```python
from build123d import *

# Parameters (mm, degrees)
SKETCH1_R                    = 2.5
BASE_FLANGE3_DEPTH           = 0.7366
SKETCHED_START               = -64
SKETCHED_BEND1_OUTLINE_W     = 0.7366
SKETCHED_BEND1_OUTLINE_H     = 65
SKETCHED_BEND1_DEPTH         = 64.108877104
SKETCHED_START_2             = 0.168203781
SKETCHED_BEND1_2_DEPTH       = 0.525916755
SKETCHED_START_3             = -0.042479464
SKETCHED_BEND1_3_DEPTH       = 1.4732
SKETCHED_START_4             = -32.5
SKETCHED_BEND1_4_DEPTH       = 65
EDGE_FLANGE1_START           = 0.7366
EDGE_FLANGE1_DEPTH           = 30.75756821
EDGE_FLANGE1_START_2         = 31.12586821
EDGE_FLANGE1_2_DEPTH         = 0.3683
EDGE_FLANGE1_3_DEPTH         = 30.38926821
SKETCH19_R                   = 1.27
SKETCH19_R_2                 = 3.3749
CUT_EXTRUDE5_DEPTH           = 112.820280988
SKETCH20_W                   = 42.572846016
SKETCH20_H                   = 16.402646855
CUT_EXTRUDE6_DEPTH           = 98.335621766
EDGE_FLANGE2_START           = 0.7366
EDGE_FLANGE2_DEPTH           = 30.75756821
EDGE_FLANGE2_START_2         = 31.12586821
EDGE_FLANGE2_2_DEPTH         = 0.3683
EDGE_FLANGE2_3_DEPTH         = 30.38926821
SKETCH27_R                   = 2.575
CUT_EXTRUDE7_DEPTH           = 10
CUT_EXTRUDE8_DEPTH           = 98.335621766
CUT_EXTRUDE8_DEPTH_BACK      = 98.335621766
SKETCH28_R                   = 1.725
SKETCH33_W                   = 30
SKETCH33_H                   = 65
SKETCH33_R                   = 2
TAB1_DEPTH                   = 0.7366
EDGE_FLANGE3_STRIP_W         = 4.4196
EDGE_FLANGE3_STRIP_H         = 0.7366
EDGE_FLANGE3_STRIP_CUT_DEPTH = 59.2634
EDGE_FLANGE3_DEPTH           = 59.2634
EDGE_FLANGE4_STRIP_W         = 4.4196
EDGE_FLANGE4_STRIP_H         = 0.7366
EDGE_FLANGE4_STRIP_CUT_DEPTH = 59.2634
EDGE_FLANGE4_DEPTH           = 59.2634


with BuildPart() as part:
    # Base-Flange3: sheet metal written as solids
    # Sketch1 → Base-Flange3 (new body)
    with BuildSketch(Plane(origin=(0, 0, 0), x_dir=(1, 0, 0), z_dir=(0, 1, 0))):
        with BuildLine():
            Line((-30.694120536, 32.5), (30.694120536, 32.5))
            Line((30.694120536, 32.5), (30.694120536, -32.5))
            Line((30.694120536, -32.5), (-30.694120536, -32.5))
            ThreePointArc((-30.694120536, -32.5), (-63.194120536, 0), (-30.694120536, 32.5))
        make_face()
        with Locations(Location((15.694120536, 0, 0), (0, 0, 270))):
            Circle(SKETCH1_R, mode=Mode.SUBTRACT)
    extrude(amount=-BASE_FLANGE3_DEPTH)

    # Sketched Bend1: read off the stored shape, not the designer's step
    # Sketched Bend1 outline → Sketched Bend1 (cut)
    with BuildSketch(Plane.YZ.offset(SKETCHED_START)):
        with Locations((-0.3683, 0)):
            Rectangle(SKETCHED_BEND1_OUTLINE_W, SKETCHED_BEND1_OUTLINE_H)
    extrude(amount=SKETCHED_BEND1_DEPTH, mode=Mode.SUBTRACT)

    # Sketched Bend1 2 outline → Sketched Bend1 2 (add)
    with BuildSketch(Plane.YZ.offset(SKETCHED_START_2)):
        with BuildLine():
            ThreePointArc((31.12586821, -32.5), (63.62586821, 0), (31.12586821, 32.5))
            Line((31.12586821, 32.5), (0, 32.5))
            Line((0, 32.5), (0, -32.5))
            Line((0, -32.5), (31.12586821, -32.5))
        make_face()
    extrude(amount=SKETCHED_BEND1_2_DEPTH)

    # Sketched Bend1 3 outline → Sketched Bend1 3 (add)
    with BuildSketch(Plane.YZ.offset(SKETCHED_START_3)):
        with BuildLine():
            ThreePointArc((31.12586821, -32.5), (63.62586821, 0), (31.12586821, 32.5))
            Line((31.12586821, 32.5), (0, 32.5))
            Line((0, 32.5), (0, -32.5))
            Line((0, -32.5), (31.12586821, -32.5))
        make_face()
    extrude(amount=SKETCHED_BEND1_3_DEPTH)

    # Sketched Bend1 4 outline → Sketched Bend1 4 (cut)
    with BuildSketch(Plane.XY.offset(SKETCHED_START_4)):
        with BuildLine():
            Line((0.694120536, 65), (0.694120536, 0.7366))
            ThreePointArc((0.694120536, 0.7366), (0.90986568, 0.215745144), (1.430720536, 0))
            Line((1.430720536, 0), (1.430720536, 65))
            Line((1.430720536, 65), (0.694120536, 65))
        make_face()
        with BuildLine():
            Line((-0.042479464, 0.7366), (-0.042479396, 65))
            Line((-0.042479396, 65), (-2, 65))
            Line((-2, 65), (-2, 0))
            Line((-2, 0), (0.108877104, 0))
            Line((0.108877104, 0), (0.108877104, -2))
            Line((0.108877104, -2), (32, -2))
            Line((32, -2), (32, -0.736599968))
            Line((32, -0.736599968), (1.430720536, -0.7366))
            ThreePointArc((1.430720536, -0.7366), (0.389010825, -0.30510971), (-0.042479464, 0.7366))
        make_face()
    extrude(amount=SKETCHED_BEND1_4_DEPTH, mode=Mode.SUBTRACT)

    # Edge-Flange1: read off the stored shape, not the designer's step
    # Edge-Flange1 outline → Edge-Flange1 (cut)
    with BuildSketch(Plane(origin=(0, 0, 0), x_dir=(1, 0, 0), z_dir=(0, 1, 0)).offset(EDGE_FLANGE1_START)):
        with BuildLine():
            ThreePointArc((0.496749161, 32.5), (0.643922463, 32.144692217), (0.694120536, 31.7634))
            Line((0.694120536, 31.7634), (0.694120536, 32.5))
            Line((0.694120536, 32.5), (0.496749161, 32.5))
        make_face()
    extrude(amount=EDGE_FLANGE1_DEPTH, mode=Mode.SUBTRACT)

    # Edge-Flange1 2 outline → Edge-Flange1 2 (cut)
    with BuildSketch(Plane(origin=(0, 0, 0), x_dir=(1, 0, 0), z_dir=(0, 1, 0)).offset(EDGE_FLANGE1_START_2)):
        with BuildLine():
            Line((-0.042479464, 31.3951), (0.694120536, 31.3951))
            Line((0.694120536, 31.3951), (0.694120536, 31.7634))
            ThreePointArc((0.694120536, 31.7634), (0.643922463, 32.144692217), (0.496749161, 32.5))
            Line((0.496749161, 32.5), (-0.042479464, 32.5))
            Line((-0.042479464, 32.5), (-0.042479464, 31.3951))
        make_face()
    extrude(amount=EDGE_FLANGE1_2_DEPTH, mode=Mode.SUBTRACT)

    # Edge-Flange1 3 outline → Edge-Flange1 3 (add)
    with BuildSketch(Plane(origin=(0, 0, 0), x_dir=(1, 0, 0), z_dir=(0, 1, 0)).offset(EDGE_FLANGE1_START)):
        with BuildLine():
            ThreePointArc((-0.779079464, 32.5), (-0.258224609, 32.284254855), (-0.042479464, 31.7634))
            Line((-0.042479464, 31.7634), (-0.042479464, 32.5))
            Line((-0.042479464, 32.5), (0.496749161, 32.5))
            ThreePointArc((0.496749161, 32.5), (-0.042479464, 33.039228625), (-0.779079464, 33.2366))
            Line((-0.779079464, 33.2366), (-65.042479464, 33.2366))
            Line((-65.042479464, 33.2366), (-65.042479464, 32.5))
            Line((-65.042479464, 32.5), (-0.779079464, 32.5))
        make_face()
    extrude(amount=EDGE_FLANGE1_3_DEPTH)

    # Sketch19 → Cut-Extrude5 (cut, through all)
    with BuildSketch(Plane.XY.offset(-32.5)):
        with Locations((-24.096722092, 26.469477583)):
            Circle(SKETCH19_R)
        with Locations((-9.310652066, 7.044552475)):
            Circle(SKETCH19_R)
        with Locations((-4.517479464, 16.06042365)):
            Circle(SKETCH19_R_2)
    extrude(amount=-CUT_EXTRUDE5_DEPTH, mode=Mode.SUBTRACT)

    # Sketch20 → Cut-Extrude6 (cut, through all)
    with BuildSketch(Plane(origin=(0.694120536, 0, 0), x_dir=(0, 0, -1), z_dir=(1, 0, 0))):
        with Locations((5.381444798, 16.092801871)):
            Rectangle(SKETCH20_W, SKETCH20_H)
    extrude(amount=-CUT_EXTRUDE6_DEPTH, mode=Mode.SUBTRACT)

    # Edge-Flange2: read off the stored shape, not the designer's step
    # Edge-Flange2 outline → Edge-Flange2 (cut)
    with BuildSketch(Plane(origin=(0, 0, 0), x_dir=(1, 0, 0), z_dir=(0, 1, 0)).offset(EDGE_FLANGE2_START)):
        with BuildLine():
            ThreePointArc((0.694120536, -31.7634), (0.643922463, -32.144692217), (0.496749161, -32.5))
            Line((0.496749161, -32.5), (0.694120536, -32.5))
            Line((0.694120536, -32.5), (0.694120536, -31.7634))
        make_face()
    extrude(amount=EDGE_FLANGE2_DEPTH, mode=Mode.SUBTRACT)

    # Edge-Flange2 2 outline → Edge-Flange2 2 (cut)
    with BuildSketch(Plane(origin=(0, 0, 0), x_dir=(1, 0, 0), z_dir=(0, 1, 0)).offset(EDGE_FLANGE2_START_2)):
        with BuildLine():
            Line((-0.042479464, -31.3951), (-0.042479464, -32.5))
            Line((-0.042479464, -32.5), (0.496749161, -32.5))
            ThreePointArc((0.496749161, -32.5), (0.643922463, -32.144692217), (0.694120536, -31.7634))
            Line((0.694120536, -31.7634), (0.694120536, -31.3951))
            Line((0.694120536, -31.3951), (-0.042479464, -31.3951))
        make_face()
    extrude(amount=EDGE_FLANGE2_2_DEPTH, mode=Mode.SUBTRACT)

    # Edge-Flange2 3 outline → Edge-Flange2 3 (add)
    with BuildSketch(Plane(origin=(0, 0, 0), x_dir=(1, 0, 0), z_dir=(0, 1, 0)).offset(EDGE_FLANGE2_START)):
        with BuildLine():
            Line((-0.779079464, -32.5), (-65.042479464, -32.5))
            Line((-65.042479464, -32.5), (-65.042479464, -33.2366))
            Line((-65.042479464, -33.2366), (-0.779079464, -33.2366))
            ThreePointArc((-0.779079464, -33.2366), (-0.042479464, -33.039228625), (0.496749161, -32.5))
            Line((0.496749161, -32.5), (-0.042479464, -32.5))
            Line((-0.042479464, -32.5), (-0.042479464, -31.7634))
            ThreePointArc((-0.042479464, -31.7634), (-0.258224609, -32.284254855), (-0.779079464, -32.5))
        make_face()
    extrude(amount=EDGE_FLANGE2_3_DEPTH)

    # Sketch27 → Cut-Extrude7 (cut)
    with BuildSketch(Plane.XY.offset(38.8834)):
        with Locations((-4.517479464, 16.06042365)):
            Circle(SKETCH27_R)
    extrude(amount=-CUT_EXTRUDE7_DEPTH, mode=Mode.SUBTRACT)

    # Sketch28 → Cut-Extrude8 (cut, two sides: drawn at the far end of the back side and taken through both)
    with BuildSketch(Plane(origin=(0.694120536, 0, 0), x_dir=(0, 0, -1), z_dir=(1, 0, 0)).offset(-CUT_EXTRUDE8_DEPTH_BACK)):
        with Locations(Location((-5.239369246, 44.083803898, 0), (0, 0, 270))):
            Circle(SKETCH28_R)
    extrude(amount=CUT_EXTRUDE8_DEPTH + CUT_EXTRUDE8_DEPTH_BACK, mode=Mode.SUBTRACT)

    # Tab1: sheet metal written as solids
    # Sketch33 → Tab1 (add)
    with BuildSketch(Plane(origin=(0, 0, 0), x_dir=(1, 0, 0), z_dir=(0, 1, 0))):
        with Locations((45.694120536, 0)):
            Rectangle(SKETCH33_W, SKETCH33_H)
        with Locations(Location((45.694120536, 17.5, 0), (0, 0, 270))):
            Circle(SKETCH33_R, mode=Mode.SUBTRACT)
        with Locations(Location((45.694120536, -17.5, 0), (0, 0, 270))):
            Circle(SKETCH33_R, mode=Mode.SUBTRACT)
    extrude(amount=-TAB1_DEPTH)

    # Edge-Flange3: sheet metal written as solids
    # Edge-Flange3 strip (on a plane across the edge) → Edge-Flange3 strip cut (cut)
    with BuildSketch(Plane(origin=(1.430720536, 0, 32.5), x_dir=(0, 0, -1), z_dir=(1, 0, 0))):
        with Locations((-0.7366, -0.3683)):
            Rectangle(EDGE_FLANGE3_STRIP_W, EDGE_FLANGE3_STRIP_H)
    extrude(amount=EDGE_FLANGE3_STRIP_CUT_DEPTH, mode=Mode.SUBTRACT)

    # Edge-Flange3 section (on a plane across the edge) → Edge-Flange3 (add)
    with BuildSketch(Plane(origin=(1.430720536, 0, 32.5), x_dir=(0, 0, -1), z_dir=(1, 0, 0))):
        with BuildLine():
            Line((0, 0.7366), (0, 30.39))
            Line((0, 30.39), (0.7366, 30.39))
            Line((0.7366, 30.39), (0.7366, 0.7366))
            ThreePointArc((0.7366, 0.7366), (0.952345145, 0.215745145), (1.4732, 0))
            Line((1.4732, 0), (1.4732, -0.7366))
            ThreePointArc((1.4732, -0.7366), (0.43149029, -0.30510971), (0, 0.7366))
        make_face()
    extrude(amount=EDGE_FLANGE3_DEPTH)

    # Edge-Flange4: sheet metal written as solids
    # Edge-Flange4 strip (on a plane across the edge) → Edge-Flange4 strip cut (cut)
    with BuildSketch(Plane(origin=(60.694120536, 0, -32.5), x_dir=(0, 0, 1), z_dir=(-1, 0, 0))):
        with Locations((-0.7366, -0.3683)):
            Rectangle(EDGE_FLANGE4_STRIP_W, EDGE_FLANGE4_STRIP_H)
    extrude(amount=EDGE_FLANGE4_STRIP_CUT_DEPTH, mode=Mode.SUBTRACT)

    # Edge-Flange4 section (on a plane across the edge) → Edge-Flange4 (add)
    with BuildSketch(Plane(origin=(60.694120536, 0, -32.5), x_dir=(0, 0, 1), z_dir=(-1, 0, 0))):
        with BuildLine():
            Line((0, 0.7366), (0, 29.6534))
            Line((0, 29.6534), (0.7366, 29.6534))
            Line((0.7366, 29.6534), (0.7366, 0.7366))
            ThreePointArc((0.7366, 0.7366), (0.952345145, 0.215745145), (1.4732, 0))
            Line((1.4732, 0), (1.4732, -0.7366))
            ThreePointArc((1.4732, -0.7366), (0.43149029, -0.30510971), (0, 0.7366))
        make_face()
    extrude(amount=EDGE_FLANGE4_DEPTH)


solid = part.part
```
For this review, take the finished solid that the model builds, in its own axes (mm). A direction names the side the tool comes from. Round coordinates to 2 decimals unless told otherwise and drop trailing zeros. Write each loop counter-clockwise with the first axis right and the second up, starting at its lowest first coordinate (ties: lowest second). Pieces come first, ordered by that corner, then holes. Notation, with made-up numbers: (22.25, 60.5) -> (29.25, 60.5) arc R24 ccw to (29.25, 84.5) -> close; hole circle Ø5 at (-29.5, 47.5). An arc over 180 degrees is marked (long way). One line per question, with ' | ' between items. Start each with the question number.
(1) Add section B-B, the plane y = 21. Write out the cut boundary in (x, z).
(2) Add section D-D, the plane z = -13. Write out the cut boundary in (x, y), plus the area to 3 significant figures.
(3) Add section A-A, the plane z = 0. Write out the cut boundary in (x, y), plus the area to 3 significant figures.
(4) Mouldability with a two-part tool opening along Y and no side actions: class faces 1 (the face through (-2.14, 15.07, 32.87)), 2 (the face through (31, 15, -31.763)), 3 (the face through (31, -0.737, 0)) as released by +Y, released by -Y, zero draft, split by the parting line, or undercut.
(5) Insertion check: P1, Ø1.2, axis at x = -30.5, z = 32.5, coming from the -Y side; P2, Ø1.5, axis at y = 52.5, z = -24.5, coming from the +X side; P3, Ø3, axis at y = 55.5, z = 4.5, coming from the -X side; P4, Ø3, axis at y = 44.08, z = 5.24, coming from the +X side. Each pin has a flat end and moves straight along its axis. Give the tip position at first contact, or say it passes through.
(6) For line 1 along X through (y, z) = (-0.4, -17.5); line 2 along Z through (x, y) = (-36, 29); line 3 along Z through (x, y) = (1.5, 9), list the stretches that pass through material, from the lowest coordinate up. Write a range as from..to.
(7) Add section C-C, the plane x = 52. Write out the cut boundary in (y, z), plus the area to 3 significant figures.
(8) Tool access review of faces 4 (the face through (-33, 16, -32.5)), 5 (the face through (31, 15, 32.5)), 6 (the face through (-24.37, 25.23, -32.86)), 7 (the face through (31, 0, 0)), 8 (the face through (31, 15, -32.5)): name each direction out of +Z, -Z, +X, -X, +Y, -Y from which nothing blocks a thin tool from reaching the whole face with its end or side.
Answer list:
1) outline: (-65.04, -33.24) -> (-0.78, -33.24) arc R1.47 ccw to (0.69, -31.76) -> (0.69, -26.67) -> (-0.04, -26.67) -> (-0.04, -31.76) arc R0.74 cw to (-0.78, -32.5) -> (-65.04, -32.5) -> close; (-65.04, 32.5) -> (-0.78, 32.5) arc R0.74 cw to (-0.04, 31.76) -> (-0.04, 15.9) -> (0.69, 15.9) -> (0.69, 31.76) arc R1.47 ccw to (-0.78, 33.24) -> (-65.04, 33.24) -> close; (1.43, -32.5) -> (60.69, -32.5) -> (60.69, -31.76) -> (1.43, -31.76) -> close; (1.43, 31.76) -> (60.69, 31.76) -> (60.69, 32.5) -> (1.43, 32.5) -> close
2) outline: (-0.04, 0.74) arc R1.47 ccw to (1.43, -0.74) -> (60.69, -0.74) -> (60.69, 0) -> (1.43, 0) arc R0.74 cw to (0.69, 0.74) -> (0.69, 7.89) -> (-0.04, 7.89) -> close; (-0.04, 24.29) -> (0.69, 24.29) -> (0.69, 60.91) -> (-0.04, 60.91) -> close | area: 77.2 mm²
3) outline: (-0.04, 0.74) arc R1.47 ccw to (1.43, -0.74) -> (13.19, -0.74) -> (13.19, 0) -> (1.43, 0) arc R0.74 cw to (0.69, 0.74) -> (0.69, 7.89) -> (-0.04, 7.89) -> close; (-0.04, 24.29) -> (0.69, 24.29) -> (0.69, 63.63) -> (-0.04, 63.63) -> close; (18.19, -0.74) -> (60.69, -0.74) -> (60.69, 0) -> (18.19, 0) -> close | area: 75.5 mm²
4) face 1: undercut | face 2: zero draft | face 3: released by -Y
5) P1: y = 0.74 | P2: x = 0.69 | P3: x = -0.04 | P4: through
6) line 1: 0.49..43.69, 47.69..60.69 | line 2: -33.24..-32.5, 32.5..33.24 | line 3: -32.5..-31.76, 31.76..32.5
7) outline: (-0.74, -31.03) arc R1.47 ccw to (0.74, -32.5) -> (29.65, -32.5) -> (29.65, -31.76) -> (0.74, -31.76) arc R0.74 cw to (0, -31.03) -> (0, 31.03) arc R0.74 cw to (0.74, 31.76) -> (30.39, 31.76) -> (30.39, 32.5) -> (0.74, 32.5) arc R1.47 ccw to (-0.74, 31.03) -> close | area: 91.4 mm²
8) face 4: -X, +Y, -Y | face 5: +Z, +X, +Y, -Y | face 6: -Z | face 7: +X, +Y | face 8: -Z, +X, +Y, -Y
